Geometry check sheet. Reference: drawing and pictorial views, mm from the part's lowest x, y, z. Give positions to 0.01 mm unless a question says otherwise; leave off trailing zeros. Write each loop counter-clockwise with the first axis right and the second up, starting at its lowest first coordinate (ties: lowest second). Pieces come first, ordered by that corner, then holes. Notation, with made-up numbers: (-10, 48) -> (42, 48) arc R7 cw to (42, 60) -> close; hole circle Ø4 at (16.25, -3.5). An arc over 180 degrees is marked (long way). Use a Markdown table: item, result. Add a question column.
1. Scan lines: probe 1 along X at (y, z) = (13.75, 2.9); probe 2 along X at (y, z) = (16, 0.7); probe 3 along Y at (x, z) = (5.25, 0.9) (3 decimals). Record each from-to range of solid material in increasing order. Write a range as [from, to].
2. Gauge pin test, flat ends, axial feed: P1, Ø3, axis at y = 15, z = 0.5, coming from the -X side; P2, Ø2, axis at y = 21.5, z = 0.5, coming from the +X side. Record the tip position at first contact, or that the pin passes through.
3. Cross-section at A-A (y = 17.75). Enter the section's corners in (x, z), then the cut area to 3 significant figures.
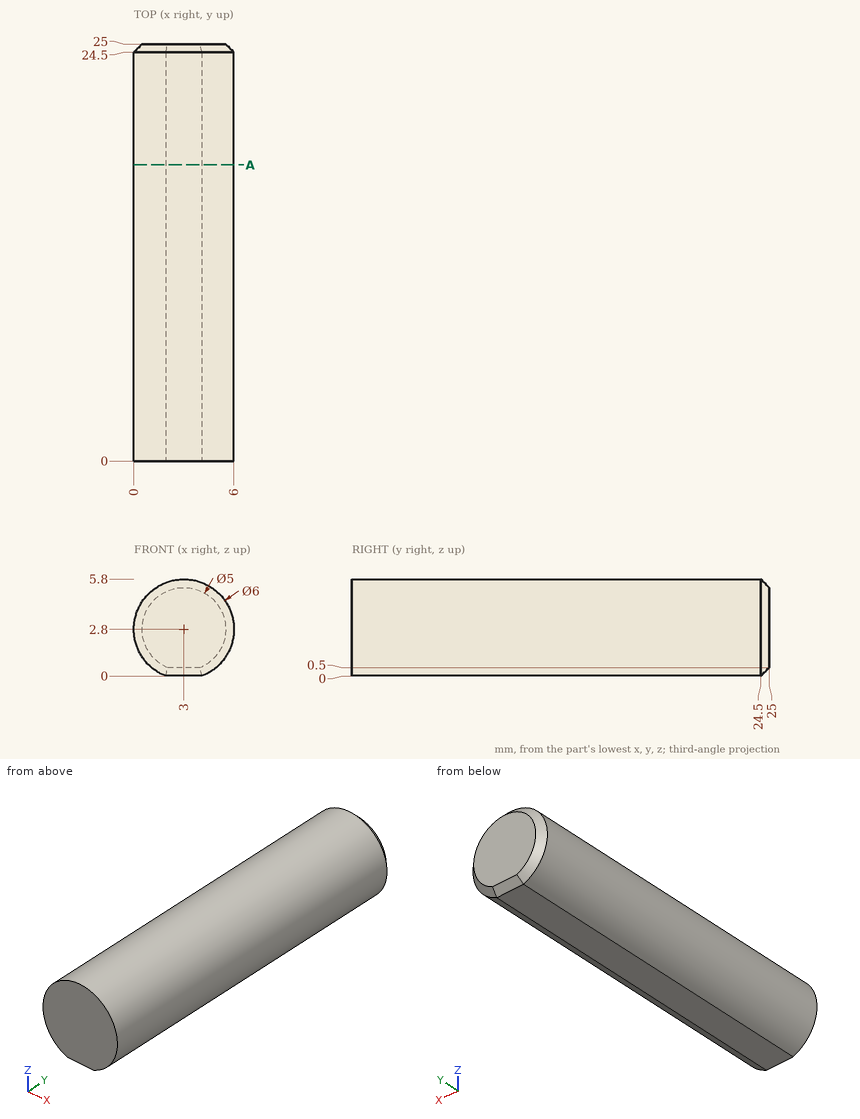
Worked answers:
| question | item | result |
|---|---|---|
| 1 | probe 1 | x = [0, 6] |
| 1 | probe 2 | x = [0.86, 5.14] |
| 1 | probe 3 | y = [0, 24.555] |
| 2 | P1 | stops at x = 0.11 |
| 2 | P2 | stops at x = 5.7 |
| 3 | outline | (1.92, 0) -> (4.08, 0) arc R3 ccw (long way) to start |
| 3 | area | 28.0 mm² |
